Work out the finished part from the listing and answer in its coordinate system (mm). Give positions to 0.01 mm unless a question says otherwise; leave off trailing zeros. Loops run counter-clockwise (first coordinate to the right, second up) from the corner with the lowest first, then second, coordinate; pieces in that order, holes last. Notation, with made-up numbers: M 47.5,17.5 L 89.5,17.5 A19 ccw 89.5,50.5 Z; hole C 25.5,40 d3. An arc over 180 degrees is marked long. Use a Markdown table: item, result.
```python
from build123d import *

# Parameters (mm, degrees)
SKETCH1_W           = 10
SKETCH1_H           = 3
BOSS_EXTRUDE1_DEPTH = 3
SKETCH4_R           = 1.1
CUT_EXTRUDE2_DEPTH  = 70.014491232


with BuildPart() as part:
    # Sketch1 → Boss-Extrude1 (new body)
    with BuildSketch(Plane.XY):
        Polygon((-65, 20), (-65, 0), (65, 0), (65, 20), (55, 20), (25, 20), (15, 20), (-15, 20), (-25, 20), (-55, 20), align=None)
        Polygon((65, 0), (-65, 0), (-65, -20), (-55, -20), (-25, -20), (-15, -20), (15, -20), (25, -20), (55, -20), (65, -20), align=None)
        with Locations((-60, 21.5)):
            Rectangle(SKETCH1_W, SKETCH1_H)
        with Locations((-20, 21.5)):
            Rectangle(SKETCH1_W, SKETCH1_H)
        with Locations((20, 21.5)):
            Rectangle(SKETCH1_W, SKETCH1_H)
        with Locations((60, 21.5)):
            Rectangle(SKETCH1_W, SKETCH1_H)
        with Locations((60, -21.5)):
            Rectangle(SKETCH1_W, SKETCH1_H)
        with Locations((20, -21.5)):
            Rectangle(SKETCH1_W, SKETCH1_H)
        with Locations((-20, -21.5)):
            Rectangle(SKETCH1_W, SKETCH1_H)
        with Locations((-60, -21.5)):
            Rectangle(SKETCH1_W, SKETCH1_H)
    extrude(amount=BOSS_EXTRUDE1_DEPTH)

    # Sketch4 → Cut-Extrude2 (cut, through all)
    with BuildSketch(Plane.XY.offset(3)):
        with Locations((-20.5, 8)):
            Circle(SKETCH4_R)
        with Locations((-20.5, -8)):
            Circle(SKETCH4_R)
        with Locations((20.5, 8)):
            Circle(SKETCH4_R)
        with Locations((20.5, -8)):
            Circle(SKETCH4_R)
        with BuildLine():
            Line((-13, 8.1), (13, 8.1))
            ThreePointArc((13, 8.1), (21.1, 0), (13, -8.1))
            Line((13, -8.1), (-13, -8.1))
            ThreePointArc((-13, -8.1), (-21.1, 0), (-13, 8.1))
        make_face()
    extrude(amount=-CUT_EXTRUDE2_DEPTH, mode=Mode.SUBTRACT)


solid = part.part
```
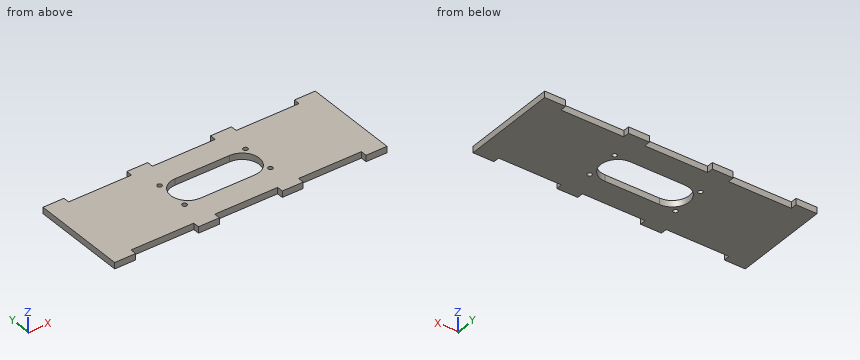
(1) A cutting plane is placed at B-B (z = 1.2). Count the separate pieces of the cut face and the enclosed holes in it, and give its area (3 significant figures).
Entries:
| item | result |
|---|---|
| separate pieces | 1 |
| enclosed holes | 5 |
| area | 4,800 mm² |
(2) A cutting plane is placed at C-C (x = -35). Write down the section's boundary in (y, z), and give its area (3 significant figures).
Entries:
| item | result |
|---|---|
| outline | M -20,0 L 20,0 L 20,3 L -20,3 Z |
| area | 120 mm² |
(3) Consider probe 1 along Y at (x, z) = (20.5, 0.6); probe 2 along Y at (x, z) = (-8.5, 2.4); probe 3 along X at (y, z) = (8.5, 0.55). Determine where each line is inside the solid, lowest interval first. Write a range as [from, to].
Entries:
| item | result |
|---|---|
| probe 1 | y = [-23, -9.1], [-6.9, -3.06], [3.06, 6.9], [9.1, 23] |
| probe 2 | y = [-20, -8.1], [8.1, 20] |
| probe 3 | x = [-65, -21.48], [-19.52, 19.52], [21.48, 65] |
(4) A cutting plane is placed at A-A (y = 0). Write down the section's boundary in (x, z).
Entries:
| item | result |
|---|---|
| outline | M -65,0 L -21.1,0 L -21.1,3 L -65,3 Z; M 21.1,0 L 65,0 L 65,3 L 21.1,3 Z |
(5) Given P1, Ø10, axis at x = -20.5, y = -14, coming from the -Z side; P2, Ø1.3, axis at x = 20.5, y = 8, coming from the +Z side; P3, Ø1.5, axis at x = -33.5, z = 1, coming from the -Y side; P4, Ø1.5, axis at x = -43.5, z = 1, coming from the +Y side, each flat-ended and moving along its own axis, determine where each tip first touches the part or whether it passes through.
Entries:
| item | result |
|---|---|
| P1 | stops at z = 0 |
| P2 | passes through |
| P3 | stops at y = -20 |
| P4 | stops at y = 20 |
